Could you check a few things on this model? Use its own coordinates, in mm. A direction names the side the tool comes from. Give positions to 0.01 mm unless a question says otherwise; leave off trailing zeros. Write each loop counter-clockwise with the first axis right and the second up, starting at its lowest first coordinate (ties: lowest second). Pieces come first, ordered by that corner, then holes. Notation, with made-up numbers: (-4, 51.25) - (13, 51.25) arc R30 ccw to (13, 80.25) - close; hole circle Ø9 at (-37, -22). An arc over 180 degrees is marked (long way). Write item = value, one per line.
Autodesk Inventor part; units mm, degrees
ref_plane "YZ Plane" through (0, 0, 0) normal (1, 0, 0) x (0, 1, 0)
ref_plane "XZ Plane" through (0, 0, 0) normal (0, 1, 0) x (-1, 0, 0)
ref_plane "XY Plane" through (0, 0, 0) normal (0, 0, 1) x (1, 0, 0)
sketch "スケッチ1" plane through (0, 0, 0) normal (0, 1, 0) x (-1, 0, 0)
  line L0 (0, 0) -> (4.5, 0)
  line L1 (4.5, 0) -> (4.5, -3)
  line L2 (4.5, -3) -> (0, -3)
  line L3 (0, -3) -> (0, 0)
  dimension "d0" = 4.5
  dimension "d1" = 3
revolve "回転1" add sketch "スケッチ1" angle 360 about axis through (0, 0, 0) along (-1, 0, 0)
sketch "スケッチ2" plane through (0, 0, 0) normal (1, 0, 0) x (0, 0, -1)
  point P0 (0, 0)
  point P1 (0, 0)
hole "穴1" at (0, 0, 0) direction (-1, 0, 0) diameter 2.459 end through all
sketch "スケッチ3" plane through (0, 0, 0) normal (1, 0, 0) x (0, 0, -1)
  circle A0 centre (0, 0) radius 3
  line L0 (3, 0) -> (-3, 0)
  line L1 (3, -0.5) -> (-3, -0.5)
  line L2 (3, 0.5) -> (-3, 0.5)
  line L3 (3, 0.5) -> (3, -0.5)
  line L4 (-3, 0.5) -> (-3, -0.5)
  point P0 (-2.958, -0.5)
  point P1 (2.958, -0.5)
  point P2 (2.958, 0.5)
  point P3 (-2.958, 0.5)
  dimension "d10" = 0.5
extrude "押し出し1" cut sketch "スケッチ3" against normal blind 1 contours L0 A0 L2 | A0 L1 L0
chamfer "面取り1" distance 0.3 angle 45 3 edges at (-4.5, 0, 3) (0, 3, 0) (0, -3, 0)
properties part number "ARU-304_5S" material "ステンレス鋼 AISI 304"
1. If we section it at B-B, the plane y = 0: Please give me the cut outline in (x, z).
Filled sheet:
outline = (-4.5, -2.7) - (-4.2, -3) - (-1, -3) - (-1, -1.23) - (-4.5, -1.23) - close; (-4.5, 1.23) - (-1, 1.23) - (-1, 3) - (-4.2, 3) - (-4.5, 2.7) - close
2. If we section it at D-D, the plane x = -1.7: Please give me the cut outline in (y, z).
Filled sheet:
outline = circle Ø6 at (0, 0); hole circle Ø2.46 at (0, 0)
3. For pin 1 (0.5 mm diameter, centred on y = 0, z = -2, fed in from +X); pin 2 (3 mm diameter, centred on y = -0.5, z = 0, fed in from -X); pin 3 (1 mm diameter, centred on x = -4, z = 1, fed in from -Y); pin 4 (2 mm diameter, centred on x = -0.5, z = -2.5, fed in from -Y), each with a flat end and sliding along its axis, tell me the tip position at first contact or that it passes through.
Filled sheet:
pin_1 = -1
pin_2 = -4.5
pin_3 = -2.96
pin_4 = -2.6
4. If we section it at C-C, the plane x = -0.7: Please give me the cut outline in (y, z).
Filled sheet:
outline = (-0.5, -2.96) - (-0.5, -1.12) arc R1.23 cw to (-0.5, 1.12) - (-0.5, 2.96) arc R3 ccw to start; (0.5, -2.96) arc R3 ccw to (0.5, 2.96) - (0.5, 1.12) arc R1.23 cw to (0.5, -1.12) - close
5. I need wall thicknesses on line 1 (Y direction, x = -1.75, z = 0); line 2 (Z direction, x = -3.3, y = -0.5). Which ranges of each line are inside material? Lowest first, please.
Filled sheet:
line_1 = -3 to -1.23, 1.23 to 3
line_2 = -2.96 to -1.12, 1.12 to 2.96
6. Which directions (+Z, -Z, +X, -X, +Y, -Y) give clear straight access to the entire face, cutting with the end or side of a thin tool? Please do faces 1 (the face through (-2.22, 0.9, -2.86)), 2 (the face through (-1, 0, 2)).
Filled sheet:
face_1 = +X, -X
face_2 = +Z, -Z, +X
7. Thinking about a two-plate mould opening in Y: for faces 3 (the face through (-2.28, -0.05, 1.23)), 4 (the face through (-0.12, 2.82, 0.06)), 5 (the face through (0, 2, 0)), 6 (the face through (-0.5, 0.5, -2.1)), which applies, pulls with the +Y half, pulls with the -Y half, needs draft (parallel to the pull), parting line crosses it, or undercut?
Filled sheet:
face_3 = undercut
face_4 = pulls with the +Y half
face_5 = needs draft
face_6 = undercut
8. If we section it at A-A, the plane z = 0: Please give me the cut outline in (x, y).
Filled sheet:
outline = (-4.5, -2.7) - (-4.2, -3) - (-0.3, -3) - (0, -2.7) - (0, -1.23) - (-4.5, -1.23) - close; (-4.5, 1.23) - (0, 1.23) - (0, 2.7) - (-0.3, 3) - (-4.2, 3) - (-4.5, 2.7) - close
